```python
from build123d import *

# Parameters (mm, degrees)
SKETCH1_R                      = 7.239
SKETCH1_R_2                    = 4.064
BOSS_EXTRUDE1_DEPTH            = 6.35
SKETCH1_3_R                    = 12.319
SKETCH1_3_R_2                  = 7.239
BOSS_EXTRUDE2_DEPTH            = 3.175
SKETCH2_R                      = 1.7
CUT_EXTRUDE1_DEPTH             = 3.175
SKETCH7_R                      = 4.8895
CUT_EXTRUDE3_DEPTH             = 3.175
CUT_EXTRUDE2_REACH             = 27.151
SKETCH5_R                      = 1.7
CUT_EXTRUDE2_DIRECTION_2_REACH = 27.151


with BuildPart() as part:
    # Sketch1 → Boss-Extrude1 (new body)
    with BuildSketch(Plane(origin=(0, 0, 0), x_dir=(1, 0, 0), z_dir=(0, 1, 0))):
        with Locations(Location((0, 0, 0), (0, 0, 270))):
            Circle(SKETCH1_R)
        with Locations(Location((0, 0, 0), (0, 0, 270))):
            Circle(SKETCH1_R_2, mode=Mode.SUBTRACT)
    extrude(amount=BOSS_EXTRUDE1_DEPTH)

    # Sketch1_3 → Boss-Extrude2 (add)
    with BuildSketch(Plane(origin=(0, 0, 0), x_dir=(1, 0, 0), z_dir=(0, 1, 0))):
        with Locations(Location((0, 0, 0), (0, 0, 270))):
            Circle(SKETCH1_3_R)
        with Locations(Location((0, 0, 0), (0, 0, 270))):
            Circle(SKETCH1_3_R_2, mode=Mode.SUBTRACT)
    extrude(amount=BOSS_EXTRUDE2_DEPTH)

    # Sketch2 → Cut-Extrude1 (cut)
    with BuildSketch(Plane(origin=(0, 3.175, 0), x_dir=(1, 0, 0), z_dir=(0, 1, 0))):
        with Locations(Location((0, 9.779, 0), (0, 0, 270))):
            Circle(SKETCH2_R)
        with Locations(Location((9.779, 0, 0), (0, 0, 270))):
            Circle(SKETCH2_R)
        with Locations(Location((0, -9.779, 0), (0, 0, 270))):
            Circle(SKETCH2_R)
        with Locations(Location((-9.779, 0, 0), (0, 0, 270))):
            Circle(SKETCH2_R)
    extrude(amount=-CUT_EXTRUDE1_DEPTH, mode=Mode.SUBTRACT)

    # Sketch7 → Cut-Extrude3 (cut)
    with BuildSketch(Plane.XZ):
        with Locations(Location((0, 0, 0), (0, 0, 270))):
            Circle(SKETCH7_R)
    extrude(amount=-CUT_EXTRUDE3_DEPTH, mode=Mode.SUBTRACT)

    # Sketch5 → Cut-Extrude2 (cut, up to next)
    with BuildSketch(Plane(origin=(-4.8895, 0, -4.8895), x_dir=(-0.7071067811865475, 0, 0.7071067811865477), z_dir=(-0.7071067811865477, 0, -0.7071067811865475)), mode=Mode.PRIVATE) as cut_extrude2_sk1:
        with Locations((0, 4.7625)):
            Circle(SKETCH5_R)
    cut_extrude2_tool1 = extrude(cut_extrude2_sk1.sketch, amount=-CUT_EXTRUDE2_REACH, mode=Mode.PRIVATE) & part.part
    add(cut_extrude2_tool1.solids().sort_by_distance((-4.8895, 4.7625, -4.8895))[0], mode=Mode.SUBTRACT)

    # Sketch5 → Cut-Extrude2 direction 2 (cut, up to next)
    with BuildSketch(Plane(origin=(-4.8895, 0, -4.8895), x_dir=(-0.7071067811865475, 0, 0.7071067811865477), z_dir=(-0.7071067811865477, 0, -0.7071067811865475)), mode=Mode.PRIVATE) as cut_extrude2_direction_2_sk1:
        with Locations((0, 4.7625)):
            Circle(SKETCH5_R)
    cut_extrude2_direction_2_tool1 = extrude(cut_extrude2_direction_2_sk1.sketch, amount=CUT_EXTRUDE2_DIRECTION_2_REACH, mode=Mode.PRIVATE) & part.part
    add(cut_extrude2_direction_2_tool1.solids().sort_by_distance((-4.8895, 4.7625, -4.8895))[0], mode=Mode.SUBTRACT)


solid = part.part
```
Check sheet for the modelled part. Datum: model origin and axes. Units: mm. A direction names the side the tool comes from. Give positions to 0.01 mm unless a question says otherwise; leave off trailing zeros. Write each loop counter-clockwise with the first axis right and the second up, starting at its lowest first coordinate (ties: lowest second). Pieces come first, ordered by that corner, then holes.
Item 1: Access from +Z, -Z, +X, -X, +Y, -Y to the whole of each face (thin tool, end or side, straight path). Record for faces 1 (the face through (-4.773, 1.565, 1.06)), 2 (the face through (2.75, 4.74, 2.99)).
Item 2: Gauge pin test, flat ends, axial feed: pin 1 (4.5 mm diameter, centred on x = 9.779, z = 0, fed in from +Y) (3 decimals); pin 2 (1 mm diameter, centred on x = 5.5, y = 5.5, fed in from +Z). Record the tip position at first contact, or that the pin passes through.
Item 3: Draft check along Y on faces 3 (the face through (-5.3, 3.175, 5.3)), 4 (the face through (-4.215, 3.064, -4.309)), 5 (the face through (0.511, 1.61, -8.158)). Enter one of: released by +Y, released by -Y, zero draft, split by the parting line, or undercut.
Item 4: Cross-section at D-D (x = 5.25). Enter the section's corners in (y, z) (3 decimals).
Item 5: Scan lines: L1, parallel to X at y = 2.4, z = 0; L2, parallel to X at y = 2.75, z = -0.5; L3, parallel to Z at x = -3.75, y = 3.5. Record each from-to range of solid material in increasing order.
Item 6: Cross-section at C-C (x = 2). Enter the section's corners in (y, z) (3 decimals).
Item 7: Cross-section at A-A (z = 0). Count the separate pieces of the cut face and the enclosed holes in it, and give its area (3 significant figures).
Item 8: Cross-section at B-B (z = 9.5). Enter the section's corners in (x, y) (3 decimals).
Report:
1. face 1: -Y
1. face 2: +Y, -Y
2. pin 1: stops at y = 3.175
2. pin 2: stops at z = 5.23
3. face 3: released by +Y
3. face 4: undercut
3. face 5: zero draft
4. outline: (0, -11.144) - (3.175, -11.144) - (3.175, -4.984) - (6.35, -4.984) - (6.35, 4.984) - (3.175, 4.984) - (3.175, 11.144) - (0, 11.144) - close
5. L1: x = -12.32 to -11.48, -8.08 to -4.89, 4.89 to 8.08, 11.48 to 12.32
5. L2: x = -12.31 to -11.4, -8.15 to -4.86, 4.86 to 8.15, 11.4 to 12.31
5. L3: z = -6.19 to -5.36, -2.14 to -1.57, 1.57 to 6.19
6. outline: (0, -12.156) - (3.175, -12.156) - (3.175, -6.957) - (6.35, -6.957) - (6.35, -3.538) - (3.175, -3.538) - (3.175, -4.462) - (0, -4.462) - close; (0, 4.462) - (3.175, 4.462) - (3.175, 3.538) - (6.35, 3.538) - (6.35, 6.957) - (3.175, 6.957) - (3.175, 12.156) - (0, 12.156) - close
7. separate pieces: 4
7. enclosed holes: 0
7. area: 45.7 mm2
8. outline: (-7.843, 0) - (-1.677, 0) - (-1.677, 3.175) - (-7.843, 3.175) - close; (1.677, 0) - (7.843, 0) - (7.843, 3.175) - (1.677, 3.175) - close
